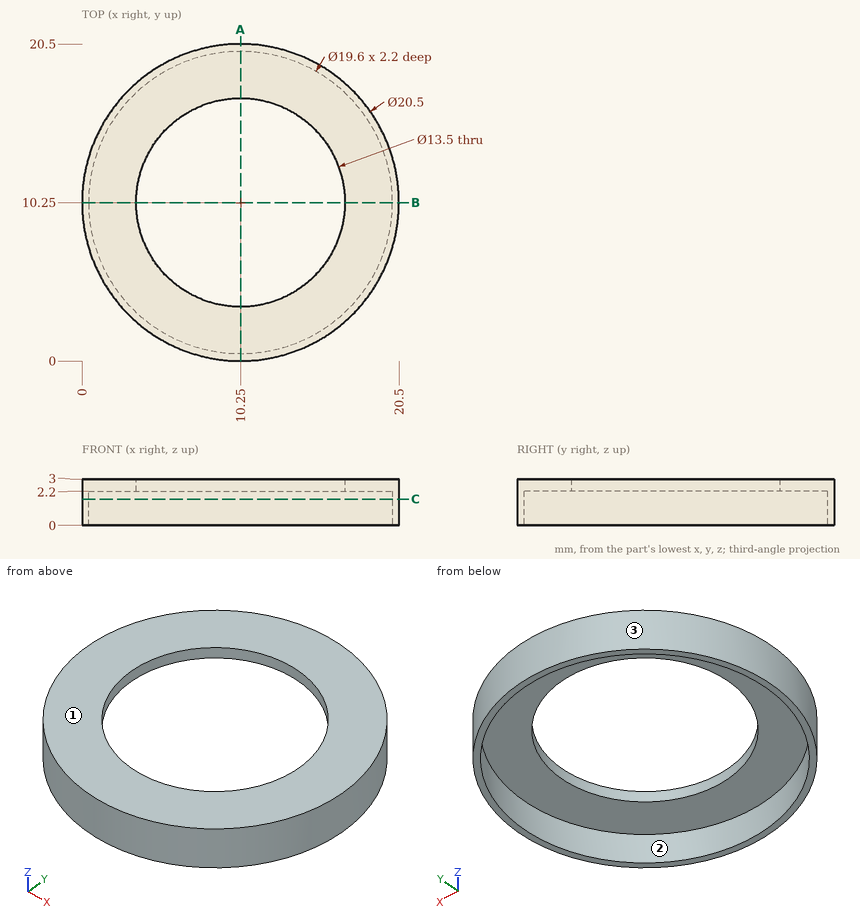
Can you work these out from the drawing? Everything is in mm from the part's minimum corner. Give positions to 0.01 mm unless a question says otherwise; leave off trailing zeros. Order: outer loops, then holes, each group sorted by start corner. A loop starts at its lowest first (then second) coordinate and runs counter-clockwise, first axis right, second up. Notation, with made-up numbers: M 11.5,2.5 L 59.5,2.5 A26 cw 59.5,25.5 Z; hole C 27,48 d11. An arc over 180 degrees is marked long. Write item = value, one per line. Start each with the question number.
Q1. We'd pull the mould along X, two halves only. Please class the marked faces 1, 2 and 3: pulls with the +X half, pulls with the -X half, needs draft (parallel to the pull), parting line crosses it, or undercut.
Q2. Will this pin go through, and if not, where does the flat tip stop? pin 1 Ø1.5 at (x, z) = (14.5, 2.5) entering from +Y.
Q3. Suppose I cut it at A-A (x = 10.25). Write out the boundary of the cut face in (y, z).
Q4. Suppose I cut it at C-C (z = 1.7). Write out the boundary of the cut face in (x, y), plus the area to 3 significant figures.
Q5. I need wall thicknesses on probe 1 along Y at (x, z) = (10.25, 2.7); probe 2 along Y at (x, z) = (10.25, 1.45). Which ranges of each line are inside material? Lowest first, please. Write a range as [from, to].
Check result:
q1.face_1 = needs draft
q1.face_2 = undercut
q1.face_3 = parting line crosses it
q2.pin_1 = 19.88
q3.outline = M 0,0 L 0.45,0 L 0.45,2.2 L 3.5,2.2 L 3.5,3 L 0,3 Z; M 17,2.2 L 20.05,2.2 L 20.05,0 L 20.5,0 L 20.5,3 L 17,3 Z
q4.outline = C 10.25,10.25 d20.5; hole C 10.25,10.25 d19.6
q4.area = 28.3 mm2
q5.probe_1 = [0, 3.5], [17, 20.5]
q5.probe_2 = [0, 0.45], [20.05, 20.5]
